Input: part model. Units: mm. Frame: model coordinates. Face numbers are marked on the shaded views. A direction names the side the tool comes from. Give positions to 0.01 mm unless a question says otherwise; leave off trailing zeros. Order: outer loops, then holes, each group sorted by start corner. A loop starts at its lowest first (then second) coordinate and runs counter-clockwise, first axis right, second up. Notation, with made-up numbers: M 75,69.5 L 102,69.5 A28 cw 102,101.5 Z; hole C -24,20.5 d1. An arc over 180 degrees is marked long. Use a Markdown table: item, result.
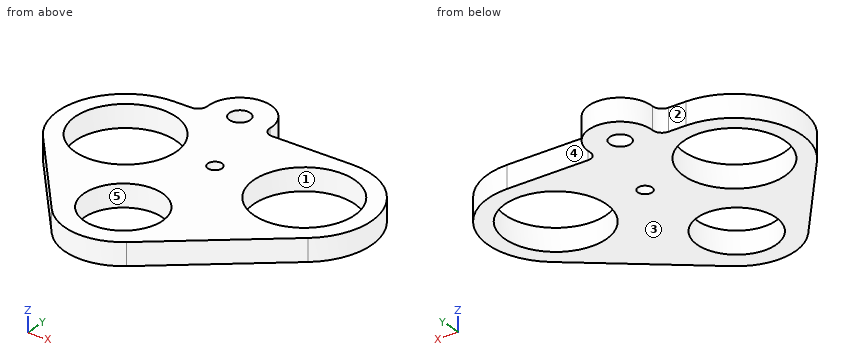
from build123d import *

# Parameters (mm, degrees)
SKETCH1_R                        = 2.9337
BOSS_EXTRUDE1_DEPTH              = 6.35
F_1_1_DIAMETER_HOLE1_D           = 28.575
F_1_1_DIAMETER_HOLE1_DEPTH       = 25.4
F_1_1_DIAMETER_HOLE1_TIP         = 8.584796094
F_7_8_0_875_DIAMETER_HOLE1_D     = 22.225
F_7_8_0_875_DIAMETER_HOLE1_DEPTH = 25.4
F_7_8_0_875_DIAMETER_HOLE1_TIP   = 6.677063629
TAP_DRILL_FOR_10_32_TAP1_D       = 4.0386
FILLET1_R                        = 2.54


with BuildPart() as part:
    # Sketch1 → Boss-Extrude1 (new body)
    with BuildSketch(Plane.XY):
        with BuildLine():
            Line((-11.605702487, 47.126767531), (-19.685, 47.126767531))
            ThreePointArc((-19.685, 47.126767531), (-36.899439748, 36.235539754), (-34.430269589, 16.015278206))
            Line((-34.430269589, 16.015278206), (-12.779233644, -10.453290749))
            ThreePointArc((-12.779233644, -10.453290749), (-1.744405346, -16.417586607), (10.297338688, -12.905228241))
            Line((10.297338688, -12.905228241), (42.996544639, 13.186119561))
            ThreePointArc((42.996544639, 13.186119561), (49.095118796, 34.371036995), (31.115, 47.126767531))
            Line((31.115, 47.126767531), (5.001702487, 47.126767531))
            ThreePointArc((5.001702487, 47.126767531), (-3.302, 59.191767531), (-11.605702487, 47.126767531))
        make_face()
        with Locations((-3.302, 50.301767531)):
            Circle(SKETCH1_R, mode=Mode.SUBTRACT)
    extrude(amount=BOSS_EXTRUDE1_DEPTH)

    # 1 (1) Diameter Hole1
    with Locations(Plane.XY.offset(6.35)):
        with Locations((-19.685, 28.076767531), (31.115, 28.076767531)):
            Hole(F_1_1_DIAMETER_HOLE1_D / 2, depth=F_1_1_DIAMETER_HOLE1_DEPTH)
            with Locations((0, 0, -(F_1_1_DIAMETER_HOLE1_DEPTH + F_1_1_DIAMETER_HOLE1_TIP / 2))):  # 118° drill point
                Cone(0, F_1_1_DIAMETER_HOLE1_D / 2, F_1_1_DIAMETER_HOLE1_TIP, mode=Mode.SUBTRACT)

    # 7/8 (0.875) Diameter Hole1
    with Locations(Plane.XY.offset(6.35)):
        with Locations((0, 0)):
            Hole(F_7_8_0_875_DIAMETER_HOLE1_D / 2, depth=F_7_8_0_875_DIAMETER_HOLE1_DEPTH)
            with Locations((0, 0, -(F_7_8_0_875_DIAMETER_HOLE1_DEPTH + F_7_8_0_875_DIAMETER_HOLE1_TIP / 2))):  # 118° drill point
                Cone(0, F_7_8_0_875_DIAMETER_HOLE1_D / 2, F_7_8_0_875_DIAMETER_HOLE1_TIP, mode=Mode.SUBTRACT)

    # Tap Drill for #10-32 Tap1 (through all)
    with Locations(Plane.XY.offset(6.35)):
        with Locations((5.715, 28.076767531)):
            Hole(TAP_DRILL_FOR_10_32_TAP1_D / 2)

    # Fillet1
    fillet1_edges = [part.edges().sort_by_distance(p)[0] for p in [
        (5.001702487, 47.126767531, 3.175),
        (-11.605702487, 47.126767531, 3.175),
    ]]
    fillet(fillet1_edges, radius=FILLET1_R)


solid = part.part
1) Cut plane A-A on x = 27.5. Return loops of the section in (y, z).
Response values:
| item | result |
|---|---|
| outline | M 0.82,0 L 14.25,0 L 14.25,6.35 L 0.82,6.35 Z; M 41.9,0 L 47.13,0 L 47.13,6.35 L 41.9,6.35 Z |
2) Cut plane D-D on z = 4.5. State how many separate pieces and enclosed holes the cut face has, and give its area (3 significant figures).
Response values:
| item | result |
|---|---|
| separate pieces | 1 |
| enclosed holes | 5 |
| area | 2,580 mm² |
3) First-contact query: pin 1 Ø23 at (x, y) = (-19.68, 28.08) entering from +Z; pin 2 Ø12 at (x, y) = (10.5, 17.5) entering from -Z; pin 3 Ø1.5 at (x, z) = (-18.5, 4.5) entering from +Y. Flat tips, straight axial feed; report the tip coordinate or a pass-through.
Response values:
| item | result |
|---|---|
| pin 1 | passes through |
| pin 2 | stops at z = 0 |
| pin 3 | stops at y = 47.13 |
4) Cut plane C-C on y = 5. Return loops of the section in (x, z).
Response values:
| item | result |
|---|---|
| outline | M -25.42,0 L -9.92,0 L -9.92,6.35 L -25.42,6.35 Z; M 9.92,0 L 32.74,0 L 32.74,6.35 L 9.92,6.35 Z |
5) Cut plane B-B on y = 25. Return loops of the section in (x, z), and give its area (3 significant figures).
Response values:
| item | result |
|---|---|
| outline | M -38.48,0 L -33.64,0 L -33.64,6.35 L -38.48,6.35 Z; M -5.73,0 L 17.16,0 L 17.16,6.35 L -5.73,6.35 Z; M 45.07,0 L 49.91,0 L 49.91,6.35 L 45.07,6.35 Z |
| area | 207 mm² |
6) Reachability of the marked faces 4 and 5 from +Z, -Z, +X, -X, +Y, -Y: full face, straight path, thin tool, end or side. Return the list, or none.
Response values:
| item | result |
|---|---|
| face 4 | +Z, -Z, +X, +Y |
| face 5 | +Z, -Z |
7) Mould query, pull axis Y, two halves, no side actions, for the marked faces 1, 2 and 3. Classes: released by +Y, released by -Y, zero draft, split by the parting line, or undercut.
Response values:
| item | result |
|---|---|
| face 1 | undercut |
| face 2 | released by +Y |
| face 3 | zero draft |
8) Material intervals for line 1 (Y direction, x = -3.5, z = 6); line 2 (X direction, y = 40, z = 1); line 3 (Y direction, x = -5, z = 1.25), sorted ascending. Write a range as from..to.
Response values:
| item | result |
|---|---|
| line 1 | y = -16.13..-10.55, 10.55..47.37, 53.23..59.19 |
| line 2 | x = -34.54..-27.56, -11.81..23.24, 38.99..45.97 |
| line 3 | y = -15.73..-9.92, 9.92..47.91, 52.69..59.03 |
